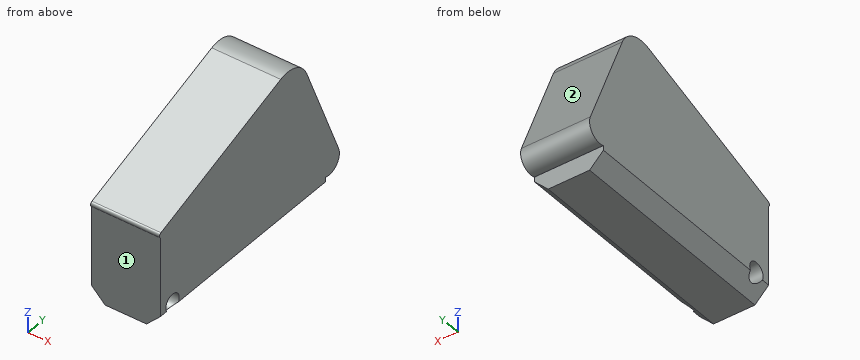
```python
from build123d import *

# Parameters (mm, degrees)
F1_DEPTH     = 25
F3_DEPTH     = 25
F5_D         = 6.5
F6_R         = 10
F7_R         = 5
F8_T1_DEPTH  = 38.943500224
F9_T1_DEPTH  = 105.7168298797
F10_T1_DEPTH = 105.7168298797


# Not quite as in the source:
# - a fillet or chamfer that OpenCascade refuses, or shapes differently, is made with other operations: its cross-section is extruded or revolved along the edge and cut away or added


with BuildPart() as f1:
    # F0 (on Right) → F1 (new body)
    with BuildSketch(Plane.YZ):
        Polygon((-44.8519773781, 0), (35.1480226219, 0), (35.1480226219, 27.3848697543), (-44.8519773781, 35), align=None)
    extrude(amount=F1_DEPTH)

    # F2 (on Right) → F3 (join)
    with BuildSketch(Plane.YZ):
        Polygon((-47.1750815473, 34.6570886492), (45.7401350141, 3.1085526571), (22.3519746214, 59.0625032783), align=None)
    extrude(amount=F3_DEPTH)

    # F5 (through all)
    with Locations(Plane(origin=(0, 0, 0), x_dir=(0, -1, 0), z_dir=(-1, 0, 0))):
        with Locations((38.9309227467, 6.3651315868)):
            Hole(F5_D / 2)

    # F6
    f6_edges = [f1.edges().sort_by_distance(p)[0] for p in [
        (12.5, 22.351975, 59.062503),
    ]]
    fillet(f6_edges, radius=F6_R)

    # F7
    f7_edges = [f1.edges().sort_by_distance(p)[0] for p in [
        (12.5, 45.740135, 3.108553),
    ]]
    fillet(f7_edges, radius=F7_R)

    # F8: fillet of radius 1 on 1 edges, made by hand

    # F8_s2 → F8_t1 (cut)
    with BuildSketch(Plane.YZ.offset(-6.971750112)):
        with BuildLine():
            ThreePointArc((-44.5437819752, 35.580728461), (-45.1967614755, 34.8143003997), (-44.8519773781, 33.8682992754))
            Line((-44.8519773781, 33.8682992754), (-44.8647654465, 33.8529218469))
            ThreePointArc((-44.8647654465, 33.8529218469), (-46.0199597269, 34.2437558604), (-47.1815118114, 34.6381505473))
            Line((-47.1815118114, 34.6381505473), (-47.1817057076, 34.6759598045))
            Line((-47.1817057076, 34.6759598045), (-44.5504061355, 35.5995996162))
            Line((-44.5504061355, 35.5995996162), (-44.5437819752, 35.580728461))
        make_face()
    extrude(amount=F8_T1_DEPTH, mode=Mode.SUBTRACT)

    # F9: chamfer of 5 on 1 edges, made by hand

    # F9_s2 → F9_t1 (cut)
    with BuildSketch(Plane.XZ.offset(-48.0064375617)):
        Polygon((20, 0), (25, 5), (25, 0), align=None)
    extrude(amount=F9_T1_DEPTH, mode=Mode.SUBTRACT)

    # F10: chamfer of 5 on 1 edges, made by hand

    # F10_s2 → F10_t1 (cut)
    with BuildSketch(Plane.XZ.offset(-48.0064375617)):
        Polygon((0, 5), (5, 0), (0, 0), align=None)
    extrude(amount=F10_T1_DEPTH, mode=Mode.SUBTRACT)


solid = f1.part
```
Geometry check sheet. Reference: the model listing, model coordinates, mm. Face numbers are marked on the shaded views. A direction names the side the tool comes from. Coordinates: 2 decimals unless noted, no trailing zeros. Order: outer loops, then holes, each group sorted by start corner. A loop starts at its lowest first (then second) coordinate and runs counter-clockwise, first axis right, second up. Notation, with made-up numbers: (79, 11) - (116, 11) arc R21 ccw to (116, 23) - close; hole circle Ø2 at (75.25, 35.5). An arc over 180 degrees is marked (long way). Answer as a JSON object with one key per item and string values. Group by question number.
Item 1: Scan lines: probe 1 along Y at (x, z) = (16.5, 4.5); probe 2 along Z at (x, y) = (2, 26); probe 3 along Z at (x, y) = (21.5, -16). Record each from-to range of solid material in increasing order.
Item 2: Tool access check on the marked faces 1 and 2. Record the directions out of +Z, -Z, +X, -X, +Y, -Y that give a thin tool (end or side, any length) a straight path to the whole face; none if there is none.
Item 3: Sectioned sample at D-D, the plane x = 4. Record the cut outline in (y, z), and give its area (3 significant figures).
Item 4: Depth check by flat-ended pin: pin 1 Ø10 at (x, y) = (18.5, 30.5) entering from +Z; pin 2 Ø3 at (y, z) = (28.5, 34) entering from -X; pin 3 Ø3 at (x, y) = (9.5, -31.5) entering from +Z; pin 4 Ø12 at (x, z) = (11, 27) entering from -Y. Enter the tip coordinate at first touch or a pass-through.
Item 5: Sectioned sample at C-C, the plane y = 34. Record the cut outline in (x, z), and give its area (3 significant figures).
Item 6: Sectioned sample at B-B, the plane x = 13.25. Record the cut outline in (y, z).
Item 7: Sectioned sample at A-A, the plane y = -37. Record the cut outline in (x, z).
Resolved:
{
 "1": {"probe 1": "-44.85 to -41.59, -36.27 to 35.15", "probe 2": "3 to 50.33", "probe 3": "1.5 to 45.6"},
 "2": {"face 1": "-Z, +X, -X, -Y", "face 2": "+Z, +X, -X, +Y"},
 "3": {"outline": "(-44.85, 1) - (35.15, 1) - (35.15, 6.71) - (35.24, 6.67) arc R5 ccw to (41.47, 13.33) - (25.99, 50.36) arc R10 ccw to (13.45, 55.94) - (-44.54, 35.58) arc R1 ccw to (-44.85, 33.87) - close; hole circle Ø6.5 at (-38.93, 6.37)", "area": "3,690 mm^2"},
 "4": {"pin 1": "z = 51.37", "pin 2": "x = 0", "pin 3": "z = 40.69", "pin 4": "y = -44.85"},
 "5": {"outline": "(0, 5) - (5, 0) - (20, 0) - (25, 5) - (25, 31.2) - (0, 31.2) - close", "area": "755 mm^2"},
 "6": {"outline": "(-44.85, 0) - (35.15, 0) - (35.15, 6.71) - (35.24, 6.67) arc R5 ccw to (41.47, 13.33) - (25.99, 50.36) arc R10 ccw to (13.45, 55.94) - (-44.54, 35.58) arc R1 ccw to (-44.85, 33.87) - close; hole circle Ø6.5 at (-38.93, 6.37)"},
 "7": {"outline": "(0, 8.98) - (25, 8.98) - (25, 38.23) - (0, 38.23) - close; (1.25, 3.75) - (5, 0) - (20, 0) - (23.75, 3.75) - close"}
}
